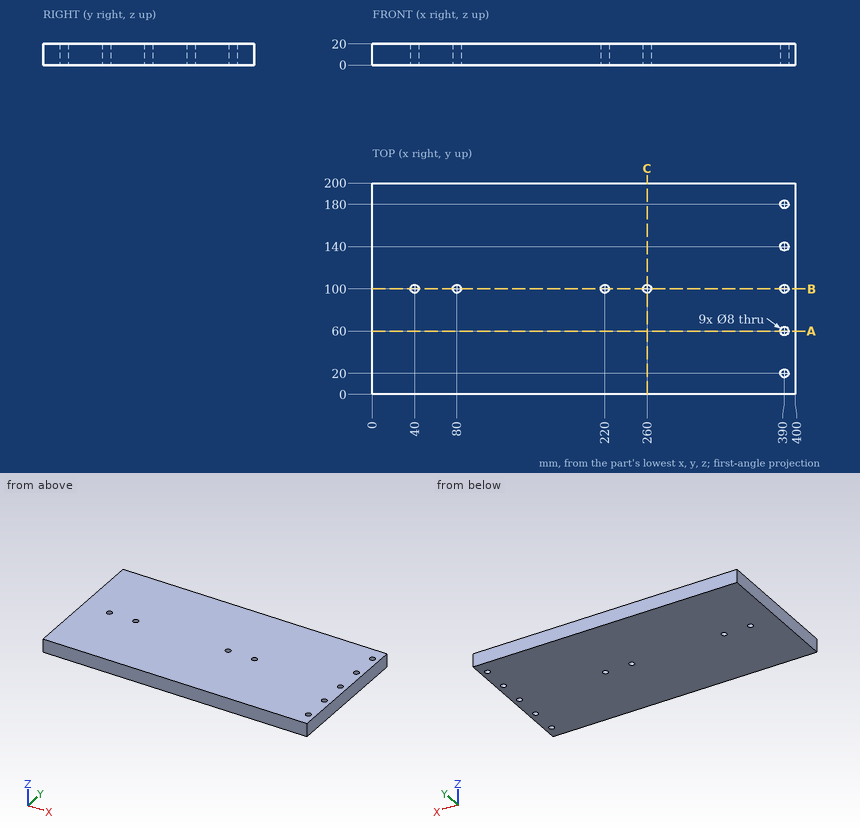
Input: dimensioned drawing with shaded views. Units: mm. Origin: part minimum x, y, z. Give positions to 0.01 mm unless a question says otherwise; leave off trailing zeros. Write each loop counter-clockwise with the first axis right and the second up, starting at its lowest first coordinate (ties: lowest second). Pieces come first, ordered by that corner, then holes. Notation, with made-up numbers: M 15,45 L 45,45 A21 ccw 45,80 Z; hole C 38.25,19.25 d4. An arc over 180 degrees is marked long. Return JSON: item names as keys, results as strings. Group by question number.
1) Pin query (flat end, axial travel): P1, Ø13, axis at x = 260, y = 100, coming from the +Z side. Return the tip coordinate at first contact, or that it passes through.
2) Cut plane A-A, the plane y = 60. Output: boundary loops of the cut face in (x, z), plus the area to 3 significant figures.
3) Cut plane B-B, the plane y = 100. Output: boundary loops of the cut face in (x, z), plus the area to 3 significant figures.
4) Cut plane C-C, the plane x = 260. Output: boundary loops of the cut face in (y, z).
5) Material intervals for line 1 along X through (y, z) = (100, 5); line 2 along Y through (x, z) = (390, 8.25); line 3 along X through (y, z) = (60, 5.25), sorted ascending. Write a range as [from, to].
Recorded:
{
 "1": {"P1": "stops at z = 20"},
 "2": {"outline": "M 0,0 L 386,0 L 386,20 L 0,20 Z; M 394,0 L 400,0 L 400,20 L 394,20 Z", "area": "7,840 mm²"},
 "3": {"outline": "M 0,0 L 36,0 L 36,20 L 0,20 Z; M 44,0 L 76,0 L 76,20 L 44,20 Z; M 84,0 L 216,0 L 216,20 L 84,20 Z; M 224,0 L 256,0 L 256,20 L 224,20 Z; M 264,0 L 386,0 L 386,20 L 264,20 Z; M 394,0 L 400,0 L 400,20 L 394,20 Z", "area": "7,200 mm²"},
 "4": {"outline": "M 0,0 L 96,0 L 96,20 L 0,20 Z; M 104,0 L 200,0 L 200,20 L 104,20 Z"},
 "5": {"line 1": "x = [0, 36], [44, 76], [84, 216], [224, 256], [264, 386], [394, 400]", "line 2": "y = [0, 16], [24, 56], [64, 96], [104, 136], [144, 176], [184, 200]", "line 3": "x = [0, 386], [394, 400]"}
}
